```python
from build123d import *

# Parameters (mm, degrees)
SKETCH1_W           = 30
SKETCH1_H           = 11.9
BOSS_EXTRUDE1_DEPTH = 8
SKETCH3_W           = 12.1
SKETCH3_H           = 11.9
CUT_EXTRUDE1_DEPTH  = 4.1
FILLET1_R           = 5


with BuildPart() as part:
    # Sketch1 → Boss-Extrude1 (new body)
    with BuildSketch(Plane(origin=(0, 0, 0), x_dir=(1, 0, 0), z_dir=(0, 1, 0))):
        Rectangle(SKETCH1_W, SKETCH1_H)
    extrude(amount=BOSS_EXTRUDE1_DEPTH)

    # Sketch3 → Cut-Extrude1 (cut)
    with BuildSketch(Plane(origin=(0, 8, 0), x_dir=(1, 0, 0), z_dir=(0, 1, 0))):
        Rectangle(SKETCH3_W, SKETCH3_H)
    extrude(amount=-CUT_EXTRUDE1_DEPTH, mode=Mode.SUBTRACT)

    # Fillet1
    fillet1_edges = [part.edges().sort_by_distance(p)[0] for p in [
        (15, 8, 0),
        (-15, 8, 0),
    ]]
    fillet(fillet1_edges, radius=FILLET1_R)


solid = part.part
```
Part model, mm, in its own coordinate system. A direction names the side the tool comes from. Coordinates: 2 decimals unless noted, no trailing zeros. Order: outer loops, then holes, each group sorted by start corner. A loop starts at its lowest first (then second) coordinate and runs counter-clockwise, first axis right, second up. Notation, with made-up numbers: (33.25, -20) -> (86.25, -20) arc R10 ccw to (86.25, -5) -> close; hole circle Ø2 at (8, 64). An arc over 180 degrees is marked (long way). Put each result on its own line as item: value. Start each with the question number.
(1) Pin check, flat tips, straight feed: pin 1 Ø1.2 at (y, z) = (7, -1.5) entering from -X; pin 2 Ø1.2 at (y, z) = (5.5, -1.5) entering from +X; pin 3 Ø2 at (y, z) = (6.5, 3) entering from -X. Stop position of each tip, or through.
(2) Band-saw the part on B-B (z = -5). Give the cut face in (x, y), then the cut area to 3 significant figures.
(3) Probe line 1 along Y through (x, z) = (0.5, -1.25); line 2 along X through (y, z) = (4.75, -3.5); line 3 along X through (y, z) = (7.25, -2.75). List the from-to ranges inside material, lowest first. Write a range as [from, to].
(4) Band-saw the part on C-C (x = 2.25). Give the cut face in (y, z), then the cut area to 3 significant figures.
(5) Which spindle directions (+Z, -Z, +X, -X, +Y, -Y) get a long thin tool onto all of the face, cutting with end or side? Do faces 1 (the face through (-6.05, 6, 0)), 2 (the face through (0, 3, 5.95)). Say none if no direction does.
(6) Band-saw the part on D-D (y = 6.5). Give the cut face in (x, z).
(7) Band-saw the part on A-A (y = 5.25). Give the cut face in (x, z), then the cut area to 3 significant figures.
Determined:
1. pin 1: stops at x = -13.67
1. pin 2: stops at x = 14.62
1. pin 3: stops at x = -14.33
2. outline: (-15, 0) -> (15, 0) -> (15, 3) arc R5 ccw to (10, 8) -> (6.05, 8) -> (6.05, 3.9) -> (-6.05, 3.9) -> (-6.05, 8) -> (-10, 8) arc R5 ccw to (-15, 3) -> close
2. area: 180 mm²
3. line 1: y = [0, 3.9]
3. line 2: x = [-14.68, -6.05], [6.05, 14.68]
3. line 3: x = [-12.63, -6.05], [6.05, 12.63]
4. outline: (0, -5.95) -> (3.9, -5.95) -> (3.9, 5.95) -> (0, 5.95) -> close
4. area: 46.4 mm²
5. face 1: +Z, -Z, +Y
5. face 2: +Z, +X, -X, +Y, -Y
6. outline: (-13.57, -5.95) -> (-6.05, -5.95) -> (-6.05, 5.95) -> (-13.57, 5.95) -> close; (6.05, -5.95) -> (13.57, -5.95) -> (13.57, 5.95) -> (6.05, 5.95) -> close
7. outline: (-14.47, -5.95) -> (-6.05, -5.95) -> (-6.05, 5.95) -> (-14.47, 5.95) -> close; (6.05, -5.95) -> (14.47, -5.95) -> (14.47, 5.95) -> (6.05, 5.95) -> close
7. area: 200 mm²
